from build123d import *

# Parameters (mm, degrees)
BOSS_EXTRUDE1_DEPTH     = 38.1
F_1_4_CLEARANCE_HOLE1_D = 6.7564
FILLET1_R               = 1.27
SKETCH23_W              = 38.1
SKETCH23_H              = 20.32
BOSS_EXTRUDE2_DEPTH     = 3.175
BOSS_EXTRUDE3_DEPTH     = 50.8
LPATTERN1_COUNT         = 2
LPATTERN1_PITCH         = 45.466
LPATTERN1_COUNT_DIR2    = 2
LPATTERN1_PITCH_DIR2    = 16.002
LPATTERN2_COUNT         = 2
LPATTERN2_PITCH         = 45.466
LPATTERN2_COUNT_DIR2    = 2
LPATTERN2_PITCH_DIR2    = 16.002
SKETCH33_R              = 2.54
CUT_EXTRUDE1_DEPTH      = 80.435936609
MIRROR7_COPY_1_SKETCH_R = 2.54
MIRROR7_COPY_1_DEPTH    = 80.435936609
SKETCH37_W              = 5.842
SKETCH37_H              = 17.272
CUT_EXTRUDE4_DEPTH      = 7.62
FILLET2_R               = 1.27


with BuildPart() as part:
    # Sketch1 → Boss-Extrude1 (new, symmetric)
    with BuildSketch(Plane(origin=(0, 0, 0), x_dir=(1, 0, 0), z_dir=(0, 1, 0))):
        with BuildLine():
            Line((0, -6.35), (66.675, -6.35))
            Line((66.675, -6.35), (66.675, 0))
            ThreePointArc((66.675, 0), (60.324997065, 6.349997065), (53.975, -5.869e-06))
            Line((53.975, -5.869e-06), (53.975, -3.81))
            Line((53.975, -3.81), (-53.975, -3.81))
            Line((-53.975, -3.81), (-53.975, 0))
            ThreePointArc((-53.975, 0), (-60.325, 6.35), (-66.675, 0))
            Line((-66.675, 0), (-66.675, -6.35))
            Line((-66.675, -6.35), (0, -6.35))
        make_face()
    extrude(amount=BOSS_EXTRUDE1_DEPTH, both=True)

    # 1/4 Clearance Hole1 (through all)
    with Locations(Plane(origin=(0, 38.1, 0), x_dir=(1, 0, 0), z_dir=(0, 1, 0))):
        with Locations((-60.325, 0)):
            f_1_4_clearance_hole1 = Hole(F_1_4_CLEARANCE_HOLE1_D / 2)

    # Mirror4: 1/4 Clearance Hole1 across plane
    add(f_1_4_clearance_hole1.mirror(Plane(origin=(0, 0, 0), x_dir=(0, 0, 1), z_dir=(1, 0, 0))), mode=Mode.SUBTRACT)

    # Fillet1
    fillet1_edges = [part.edges().sort_by_distance(p)[0] for p in [
        (-53.975, 0, 3.81),
        (53.975, 0, 3.81),
    ]]
    fillet(fillet1_edges, radius=FILLET1_R)

    # Sketch23 → Boss-Extrude2 (add)
    with BuildSketch(Plane(origin=(0, 38.1, 0), x_dir=(1, 0, 0), z_dir=(0, 1, 0))):
        with Locations((-22.733, 6.35)):
            Rectangle(SKETCH23_W, SKETCH23_H)
    boss_extrude2 = extrude(amount=-BOSS_EXTRUDE2_DEPTH)

    # Sketch24 → Boss-Extrude3 (add)
    with BuildSketch(Plane.XZ.offset(-34.925)):
        Polygon((-35.941, 3.81), (-41.783, 3.81), (-41.783, -16.51), (-22.733, -16.51), (-22.733, -13.462), (-35.941, -13.462), align=None)
        Polygon((-22.733, -13.462), (-22.733, -16.51), (-3.683, -16.51), (-3.683, 3.81), (-9.525, 3.81), (-9.525, -13.462), align=None)
    boss_extrude3 = extrude(amount=BOSS_EXTRUDE3_DEPTH)

    # Mirror5: Boss-Extrude2, Boss-Extrude3 across plane
    add(boss_extrude2.mirror(Plane(origin=(0, 0, 0), x_dir=(0, 0, 1), z_dir=(1, 0, 0))))
    add(boss_extrude3.mirror(Plane(origin=(0, 0, 0), x_dir=(0, 0, 1), z_dir=(1, 0, 0))))

    # Sketch30 → Ø1.0 mm Dowel Holes1 (revolve, cut)
    with BuildSketch(Plane(origin=(-6.604, 30.48, 6.35), x_dir=(0, -1, 0), z_dir=(1, 0, 0))):
        Polygon((0, 0), (0, 6.831753069), (2.05, 5.5999888), (2.05, 0), align=None)
    f_1_0_mm_dowel_holes1 = revolve(axis=Axis((-6.604, 30.48, 12.7), (0, 0, -1)), mode=Mode.SUBTRACT)

    # LPattern1: 1.0 mm Dowel Holes1 2 × 2
    with Locations(*[(i * LPATTERN1_PITCH, -j * LPATTERN1_PITCH_DIR2, 0) for i in range(LPATTERN1_COUNT) for j in range(LPATTERN1_COUNT_DIR2) if (i, j) != (0, 0)]):
        add(f_1_0_mm_dowel_holes1, mode=Mode.SUBTRACT)

    # Sketch32 → Ø1.0 mm Dowel Holes2 (revolve, cut)
    with BuildSketch(Plane(origin=(6.604, 4.318, 6.35), x_dir=(0, -1, 0), z_dir=(1, 0, 0))):
        Polygon((0, 0), (0, 6.831753069), (2.05, 5.5999888), (2.05, 0), align=None)
    f_1_0_mm_dowel_holes2 = revolve(axis=Axis((6.604, 4.318, 12.7), (0, 0, -1)), mode=Mode.SUBTRACT)

    # LPattern2: 1.0 mm Dowel Holes2 2 × 2
    with Locations(*[(-i * LPATTERN2_PITCH, -j * LPATTERN2_PITCH_DIR2, 0) for i in range(LPATTERN2_COUNT) for j in range(LPATTERN2_COUNT_DIR2) if (i, j) != (0, 0)]):
        add(f_1_0_mm_dowel_holes2, mode=Mode.SUBTRACT)

    # Sketch33 → Cut-Extrude1 (cut, through all)
    with BuildSketch(Plane(origin=(0, 0, 3.81), x_dir=(-1, 0, 0), z_dir=(0, 0, -1))):
        with Locations((-30.353, -19.685)):
            Circle(SKETCH33_R)
    cut_extrude1 = extrude(amount=-CUT_EXTRUDE1_DEPTH, mode=Mode.SUBTRACT)

    # Mirror6: Cut-Extrude1 across plane
    add(cut_extrude1.mirror(Plane.ZY.offset(-22.733)), mode=Mode.SUBTRACT)

    # Mirror7: Cut-Extrude1 across plane
    add(cut_extrude1.mirror(Plane(origin=(0, 0, 0), x_dir=(0, 0, 1), z_dir=(1, 0, 0))), mode=Mode.SUBTRACT)

    # Mirror7 copy 1 sketch → Mirror7 copy 1 (cut, through all)
    with BuildSketch(Plane(origin=(-45.466, 0, 3.81), x_dir=(-1, 0, 0), z_dir=(0, 0, -1))):
        with Locations((-30.353, -19.685)):
            Circle(MIRROR7_COPY_1_SKETCH_R)
    extrude(amount=-MIRROR7_COPY_1_DEPTH, mode=Mode.SUBTRACT)

    # Sketch37 → Cut-Extrude4 (cut)
    with BuildSketch(Plane.XZ.offset(15.875)):
        with Locations((38.862, -4.826)):
            Rectangle(SKETCH37_W, SKETCH37_H)
    cut_extrude4 = extrude(amount=-CUT_EXTRUDE4_DEPTH, mode=Mode.SUBTRACT)

    # Mirror11: Cut-Extrude4 across plane
    add(cut_extrude4.mirror(Plane.ZY.offset(-16.129)), mode=Mode.SUBTRACT)

    # Fillet2
    fillet2_edges = [part.edges().sort_by_distance(p)[0] for p in [
        (9.525, -15.875, -4.826),
        (41.783, 14.9225, 3.81),
        (35.941, -8.255, -4.826),
        (-3.683, 14.9225, 3.81),
        (-9.525, -8.255, -4.826),
        (-41.783, 11.1125, 3.81),
        (-41.783, 11.1125, -16.51),
        (-3.683, 11.1125, -16.51),
        (-35.941, -15.875, -4.826),
        (41.783, 11.1125, -16.51),
        (3.683, 11.1125, 3.81),
        (3.683, 11.1125, -16.51),
    ]]
    fillet(fillet2_edges, radius=FILLET2_R)


solid = part.part
The listing builds one solid part. Answer for the finished solid, in the listing's coordinates (mm). A direction names the side the tool comes from. Round coordinates to 2 decimals unless told otherwise and drop trailing zeros. Write each loop counter-clockwise with the first axis right and the second up, starting at its lowest first coordinate (ties: lowest second). Pieces come first, ordered by that corner, then holes. Notation, with made-up numbers: (-5.5, -31.5) - (0.5, -31.5) arc R25 cw to (0.5, -3.5) - close; hole circle Ø5 at (0, 55.25). An arc over 180 degrees is marked (long way). Use a Markdown table: item, result. Add a question column.
1. A tool of negligible diameter and unlimited length cuts with its end or side. For faces 1 (the face through (53.975, 1, 1)), 2 (the face through (-1, 1, 6.35)), 3 (the face through (-23, 34.925, -5)), 4 (the face through (-66.675, 1, 3)), 5 (the face through (-40.895, 4.585, 3.589)), from which of +Z, -Z, +X, -X, +Y, -Y can it reach the whole face along a straight path? Write none if from no direction.
2. Flat-ended cylindrical pins translate along their axes: P1, Ø2, axis at x = -1.5, z = -12.5, coming from the +Y side; P2, Ø6, axis at x = 15.113, y = -19.685, coming from the +Z side; P3, Ø6.5, axis at x = -15.113, y = -19.685, coming from the -Z side; P4, Ø5.5, axis at y = 2, z = -5.5, coming from the +X side. Find the tip coordinate at first contact, or state that the pin passes through.
3. The part is cut by section C-C (y = 8). Give the number of separate pieces and of enclosed holes in the cut face, and give its area (3 significant figures).
4. The part is cut by section B-B (x = -24.5). Write down the section's boundary in (y, z) (3 decimals).
5. For a pull along Y with two mould halves and no side action, classify faces 6 (the face through (-6, -8.255, -5)), 7 (the face through (-38.514, 4.395, -0.268)), 8 (the face through (-1, 38.1, 5)) as +Y half, -Y half, draft (parallel to the pull), parting line (faces both ways), or undercut.
6. The part is cut by section A-A (z = -12). Write down the section's boundary in (x, y) (3 decimals), and give its area (3 significant figures).
7. Consider line 1 (X direction, y = 30.48, z = 4.4) (3 decimals); line 2 (X direction, y = -9, z = 1) (3 decimals); line 3 (X direction, y = -3, z = -11) (3 decimals). Determine where each line is inside the solid, lowest interval first.
Reported:
| question | item | result |
|---|---|---|
| 1 | face 1 | -Z, +Y, -Y |
| 1 | face 2 | +Z, +X, -X, +Y, -Y |
| 1 | face 3 | -Y |
| 1 | face 4 | +Z, -Z, -X, +Y, -Y |
| 1 | face 5 | +Z |
| 2 | P1 | through |
| 2 | P2 | z = 6.35 |
| 2 | P3 | z = 3.81 |
| 2 | P4 | x = 66.05 |
| 3 | separate pieces | 1 |
| 3 | enclosed holes | 4 |
| 3 | area | 1,130 mm^2 |
| 4 | outline | (-38.1, 3.81) - (34.925, 3.81) - (34.925, -13.462) - (-15.875, -13.462) - (-15.875, -16.51) - (38.1, -16.51) - (38.1, 6.35) - (-38.1, 6.35) - close |
| 5 | face 6 | -Y half |
| 5 | face 7 | undercut |
| 5 | face 8 | +Y half |
| 6 | outline | (-41.783, -15.875) - (-37.211, -15.875) arc R1.27 ccw to (-35.941, -14.605) - (-35.941, 34.925) - (-9.525, 34.925) - (-9.525, -6.985) arc R1.27 ccw to (-8.255, -8.255) - (-3.683, -8.255) - (-3.683, 38.1) - (-41.783, 38.1) - close; (3.683, -15.875) - (8.255, -15.875) arc R1.27 ccw to (9.525, -14.605) - (9.525, 34.925) - (35.941, 34.925) - (35.941, -6.985) arc R1.27 ccw to (37.211, -8.255) - (41.783, -8.255) - (41.783, 38.1) - (3.683, 38.1) - close |
| 6 | area | 1,340 mm^2 |
| 7 | line 1 | -66.675 to -8.654, -4.554 to 36.812, 40.912 to 66.675 |
| 7 | line 2 | -66.675 to -63.552, -57.098 to -53.975, -41.783 to -35.941, 3.683 to 9.525, 53.975 to 57.098, 63.552 to 66.675 |
| 7 | line 3 | -41.783 to -35.941, -9.525 to -3.683, 3.683 to 9.525, 35.941 to 41.783 |
